Autodesk Inventor part; units mm, degrees
ref_plane "rail25_to_dummy_XY" through (0, 0, 360) normal (0, 0, 1) x (1, 0, 0)
ref_plane "rail25_to_dummy_YZ" through (0, 0, 360) normal (1, 0, 0) x (0, 1, 0)
ref_plane "rail25_to_dummy_ZX" through (0, 0, 360) normal (0, 1, 0) x (0, 0, 1)
sketch "Sketch_1" plane through (0, 0, 0) normal (0, 0, 1) x (1, 0, 0)
  arc A0 (-12.5, 1) -> (-11.5, 0) centre (-11.5, 1) ccw
  line L0 (-11.5, 0) -> (11.5, 0)
  arc A1 (11.5, 0) -> (12.5, 1) centre (11.5, 1) ccw
  line L1 (12.5, 1) -> (12.5, 7.5)
  arc A2 (12.5, 7.5) -> (11.5, 8.5) centre (11.5, 7.5) ccw
  line L2 (11.5, 8.5) -> (9.5, 8.5)
  arc A3 (9.5, 8.5) -> (8.6036, 7.9432) centre (9.5, 7.5) ccw
  arc A4 (8.5, 3.4087) -> (8.6036, 7.9432) centre (7.5, 5.7) ccw
  line L3 (8.5, 3.4087) -> (8.5, 2.5)
  arc A5 (8, 2) -> (8.5, 2.5) centre (8, 2.5) ccw
  line L4 (8, 2) -> (-8, 2)
  arc A6 (-8.5, 2.5) -> (-8, 2) centre (-8, 2.5) ccw
  line L5 (-8.5, 2.5) -> (-8.5, 3.4087)
  arc A7 (-8.6036, 7.9432) -> (-8.5, 3.4087) centre (-7.5, 5.7) ccw
  arc A8 (-8.6036, 7.9432) -> (-9.5, 8.5) centre (-9.5, 7.5) ccw
  line L6 (-9.5, 8.5) -> (-11.5, 8.5)
  arc A9 (-11.5, 8.5) -> (-12.5, 7.5) centre (-11.5, 7.5) ccw
  line L7 (-12.5, 7.5) -> (-12.5, 1)
extrude "Extrusion1" add sketch "Sketch_1" along normal blind 720
sketch "Sketch_2" plane through (0, 0, 40) normal (0, 0, 1) x (1, 0, 0)
  line L0 (0, 0) -> (0, 2)
  line L1 (0, 2) -> (4.25, 2)
  line L2 (4.25, 2) -> (2.25, 0)
  line L3 (2.25, 0) -> (0, 0)
  line L4 (0, 0) -> (0, 2)
revolve "Revolution1" cut sketch "Sketch_2" angle 360 about axis through (0, 0, 40) along (0, -1, 0)
pattern_linear "Rectangular Pattern1" count 9 spacing 80 along (0, 0, 1) of "Revolution1"
sketch "Sketch_4" plane through (0, 2, 0) normal (0, 1, 0) x (1, 0, 0)
  circle A0 centre (0, -3) radius 5
extrude "Extrusion2" add sketch "Sketch_4" along normal blind 5
sketch "Sketch_5" plane through (0, 2, 0) normal (0, 1, 0) x (1, 0, 0)
  circle A0 centre (0, -717) radius 5
extrude "Extrusion3" add sketch "Sketch_5" along normal blind 5
ref_plane "rail25_to_dummy_XY" through (0, 0, 360) normal (0, 0, 1) x (1, 0, 0)
ref_plane "rail25_to_dummy_YZ" through (0, 0, 360) normal (1, 0, 0) x (0, 1, 0)
ref_plane "rail25_to_dummy_ZX" through (0, 0, 360) normal (0, 1, 0) x (0, 0, 1)
ref_plane "to_slider_XY" through (0, 12, 360) normal (0, 0, 1) x (1, 0, 0)
ref_plane "to_slider_YZ" through (0, 12, 360) normal (1, 0, 0) x (0, 1, 0)
ref_plane "to_slider_ZX" through (0, 12, 360) normal (0, 1, 0) x (0, 0, 1)
properties part number "RSRR25-720"
The listing builds one solid part. Answer for the finished solid, in the listing's coordinates (mm). Give positions to 0.01 mm unless a question says otherwise; leave off trailing zeros. Write each loop counter-clockwise with the first axis right and the second up, starting at its lowest first coordinate (ties: lowest second). Pieces come first, ordered by that corner, then holes. Notation, with made-up numbers: (-7, 17) - (6, 17) arc R24 cw to (6, 42) - close; hole circle Ø5 at (83, -33.75). An arc over 180 degrees is marked (long way). Use a Markdown table: item, result.
1. Each of these flat-tipped pins is pushed along its axis until it touches: P1, Ø11, axis at x = 1.5, z = 715, coming from the +Y side; P2, Ø2.5, axis at x = -5, y = 5, coming from the +Z side; P3, Ø1, axis at x = -1, z = 721, coming from the -Y side. Where does it stop, or does it pass through?
Values follow:
| item | result |
|---|---|
| P1 | stops at y = 7 |
| P2 | stops at z = 720.31 |
| P3 | stops at y = 2 |
2. Section A-A on z = 51 is taken. Write down the section's boundary in (x, y), plus the area to 3 significant figures.
Values follow:
| item | result |
|---|---|
| outline | (-12.5, 1) arc R1 ccw to (-11.5, 0) - (11.5, 0) arc R1 ccw to (12.5, 1) - (12.5, 7.5) arc R1 ccw to (11.5, 8.5) - (9.5, 8.5) arc R1 ccw to (8.6, 7.94) arc R2.5 cw to (8.5, 3.41) - (8.5, 2.5) arc R0.5 cw to (8, 2) - (-8, 2) arc R0.5 cw to (-8.5, 2.5) - (-8.5, 3.41) arc R2.5 cw to (-8.6, 7.94) arc R1 ccw to (-9.5, 8.5) - (-11.5, 8.5) arc R1 ccw to (-12.5, 7.5) - close |
| area | 90.9 mm² |
3. For a pull along Z with two mould halves and no side action, classify faces 1 (the flat face through (0, 2, 355)), 2 (the flat face through (0, 0, 355)) as released by +Z, released by -Z, zero draft, split by the parting line, or undercut.
Values follow:
| item | result |
|---|---|
| face 1 | undercut |
| face 2 | zero draft |
4. Find the intervals of material crossed by probe 1 along X at (y, z) = (6.5, 577.5); probe 2 along X at (y, z) = (6, 500); probe 3 along Y at (x, z) = (-6.25, 66), in increasing order. Write a range as from..to.
Values follow:
| item | result |
|---|---|
| probe 1 | x = -12.5..-9.87, 9.87..12.5 |
| probe 2 | x = -12.5..-9.98, 9.98..12.5 |
| probe 3 | y = 0..2 |
